Can you work these out from the model? Positions are in its coordinate system, mm. Round coordinates to 2 decimals unless told otherwise and drop trailing zeros. Order: outer loops, then holes, each group sorted by start corner. A loop starts at its lowest first (then second) coordinate and runs counter-clockwise, first axis right, second up.
Autodesk Inventor part; units mm, degrees
ref_plane "YZ Plane" through (0, 0, 0) normal (1, 0, 0) x (0, 1, 0)
ref_plane "XZ Plane" through (0, 0, 0) normal (0, 1, 0) x (-1, 0, 0)
ref_plane "XY Plane" through (0, 0, 0) normal (0, 0, 1) x (1, 0, 0)
sketch "Sketch1" plane through (0, 0, 0) normal (0, 0, 1) x (1, 0, 0)
  line L0 (-95, -31.5) -> (95, -31.5)
  line L1 (95, -31.5) -> (95, 31.5)
  line L2 (95, 31.5) -> (-95, 31.5)
  line L3 (-95, 31.5) -> (-95, -31.5)
  line L4 (-95, -31.5) -> (95, 31.5) construction
  line L5 (95, -31.5) -> (-95, 31.5) construction
  point P0 (0, 0)
  dimension "d0" = 190
  dimension "d1" = 63
extrude "Extrusion1" add sketch "Sketch1" along normal blind 3
sketch "Sketch2" plane through (0, 0, 3) normal (0, 0, 1) x (1, 0, 0)
  line L0 (-95, 31.5) -> (-95, -31.5)
  line L1 (-95, -31.5) -> (-92, -31.5)
  line L2 (-92, -31.5) -> (-92, -1.5)
  line L3 (-92, -1.5) -> (-95, -1.5)
  line L4 (-95, -1.5) -> (-95, -31.5)
  line L5 (-92, -31.5) -> (-72, -31.5)
  line L6 (-72, -31.5) -> (-72, -28.5)
  line L7 (-72, -28.5) -> (-92, -28.5)
  line L8 (-92, -28.5) -> (-92, -31.5)
  line L9 (-95, -31.5) -> (95, -31.5)
  line L10 (-62, -31.5) -> (-47, -31.5)
  line L11 (-47, -31.5) -> (-47, -28.5)
  line L12 (-47, -28.5) -> (-62, -28.5)
  line L13 (-62, -28.5) -> (-62, -31.5)
  line L14 (-37, -31.5) -> (-22, -31.5)
  line L15 (-22, -31.5) -> (-22, -28.5)
  line L16 (-22, -28.5) -> (-37, -28.5)
  line L17 (-37, -28.5) -> (-37, -31.5)
  line L18 (-12, -31.5) -> (3, -31.5)
  line L19 (3, -31.5) -> (3, -28.5)
  line L20 (3, -28.5) -> (-12, -28.5)
  line L21 (-12, -28.5) -> (-12, -31.5)
  line L22 (13, -31.5) -> (28, -31.5)
  line L23 (28, -31.5) -> (28, -28.5)
  line L24 (28, -28.5) -> (13, -28.5)
  line L25 (13, -28.5) -> (13, -31.5)
  line L26 (38, -31.5) -> (53, -31.5)
  line L27 (53, -31.5) -> (53, -28.5)
  line L28 (53, -28.5) -> (38, -28.5)
  line L29 (38, -28.5) -> (38, -31.5)
  line L30 (95, -31.5) -> (92, -31.5)
  line L31 (92, -31.5) -> (92, -1.5)
  line L32 (92, -1.5) -> (95, -1.5)
  line L33 (95, -1.5) -> (95, -31.5)
  line L34 (92, -31.5) -> (63, -31.5)
  line L35 (63, -31.5) -> (63, -28.5)
  line L36 (63, -28.5) -> (92, -28.5)
  line L37 (92, -28.5) -> (92, -31.5)
  point P0 (0, 0)
  dimension "d4" = 3
  dimension "d5" = 30
  dimension "d7" = 20
  dimension "d8" = 3
  dimension "d9" = 15
  dimension "d10" = 15
  dimension "d11" = 15
  dimension "d12" = 15
  dimension "d13" = 15
  dimension "d14" = 10
  dimension "d15" = 10
  dimension "d16" = 10
  dimension "d17" = 10
  dimension "d18" = 10
  dimension "d20" = 3
  dimension "d21" = 30
  dimension "d22" = 10
extrude "Extrusion2" cut sketch "Sketch2" against normal through all
sketch "Sketch3" plane through (0, 0, 3) normal (0, 0, 1) x (1, 0, 0)
  line L0 (95, 31.5) -> (-95, 31.5)
  line L1 (-15, 31.5) -> (55, 31.5)
  line L2 (55, 31.5) -> (55, 28.5)
  line L3 (55, 28.5) -> (-15, 28.5)
  line L4 (-15, 28.5) -> (-15, 31.5)
  line L5 (95, -1.5) -> (95, 31.5)
  line L6 (-75, 31.5) -> (-55, 31.5)
  line L7 (-55, 31.5) -> (-55, 28.5)
  line L8 (-55, 28.5) -> (-75, 28.5)
  line L9 (-75, 28.5) -> (-75, 31.5)
  line L10 (-95, 31.5) -> (-95, -1.5)
  point P0 (0, 0)
  dimension "d25" = 3
  dimension "d26" = 40
  dimension "d27" = 70
  dimension "d28" = 20
  dimension "d29" = 20
extrude "Extrusion3" cut sketch "Sketch3" against normal through all
equation "\"d10\" = d9"
equation "\"d11\" = d10"
equation "\"d12\" = d11"
equation "\"d13\" = d12"
equation "\"d15\" = d14"
equation "\"d16\" = d15"
equation "\"d17\" = d16"
equation "\"d18\" = d16"
equation "\"d22\" = d14"
properties part number "back"
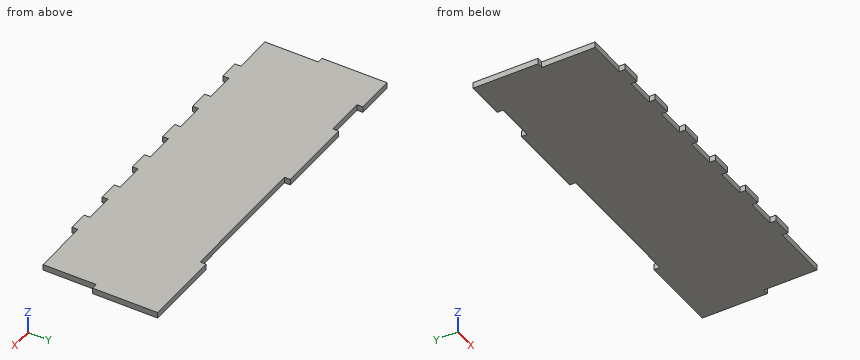
(1) I want a section at A-A, the plane y = -25.5. List the corners of the cut face in (x, z) for me.
(2) I'm going to push flat-ended pins straight in: pin 1 Ø0.9 at (y, z) = (-30.5, 2) entering from +X; pin 2 Ø1.5 at (y, z) = (-17, 1) entering from -X; pin 3 Ø1.5 at (x, z) = (-56, 1.5) entering from -Y. Where does each tip first touch, or does it pass through?
(3) I want a section at B-B, the plane x = -60. List the corners of the cut face in (y, z) for me, plus the area to 3 significant figures.
(4) Please list where these lines run through material, in increasing order: probe 1 along X at (y, z) = (29.5, 0.75); probe 2 along Y at (x, z) = (22, 1.65); probe 3 along Y at (x, z) = (28.5, 1.9).
Ans:
1. outline: (-92, 0) - (92, 0) - (92, 3) - (-92, 3) - close
2. pin 1: stops at x = 63
2. pin 2: stops at x = -92
2. pin 3: stops at y = -28.5
3. outline: (-28.5, 0) - (28.5, 0) - (28.5, 3) - (-28.5, 3) - close
3. area: 171 mm2
4. probe 1: x = -95 to -75, -55 to -15, 55 to 95
4. probe 2: y = -28.5 to 28.5
4. probe 3: y = -31.5 to 28.5
